from build123d import *

# Parameters (mm, degrees)
SKETCH1_W           = 9.525
SKETCH1_H           = 9.525
BOSS_EXTRUDE1_DEPTH = 5.1816
SKETCH2_R           = 3.175
BOSS_EXTRUDE2_DEPTH = 6.35
BOSS_EXTRUDE3_DEPTH = 0.762
SKETCH4_R           = 1.5875
BOSS_EXTRUDE4_DEPTH = 6.35
CUT_EXTRUDE1_DEPTH  = 4.826
SKETCH6_R           = 0.254
BOSS_EXTRUDE5_DEPTH = 5.969


with BuildPart() as part:
    # Sketch1 → Boss-Extrude1 (new body)
    with BuildSketch(Plane(origin=(0, 0, 0), x_dir=(1, 0, 0), z_dir=(0, 1, 0))):
        Rectangle(SKETCH1_W, SKETCH1_H)
    extrude(amount=-BOSS_EXTRUDE1_DEPTH)

    # Sketch2 → Boss-Extrude2 (add)
    with BuildSketch(Plane(origin=(0, 0, 0), x_dir=(1, 0, 0), z_dir=(0, 1, 0))):
        Circle(SKETCH2_R)
    extrude(amount=BOSS_EXTRUDE2_DEPTH)

    # Sketch3 → Boss-Extrude3 (add)
    with BuildSketch(Plane(origin=(0, 0, 0), x_dir=(1, 0, 0), z_dir=(0, 1, 0))):
        with BuildLine():
            Line((-4.7625, 0.381), (-4.7625, -0.381))
            ThreePointArc((-4.7625, -0.381), (-4.3815, 0), (-4.7625, 0.381))
        make_face()
    extrude(amount=BOSS_EXTRUDE3_DEPTH)

    # Sketch4 → Boss-Extrude4 (add)
    with BuildSketch(Plane(origin=(0, 6.35, 0), x_dir=(1, 0, 0), z_dir=(0, 1, 0))):
        Circle(SKETCH4_R)
    extrude(amount=BOSS_EXTRUDE4_DEPTH)

    # Sketch5 → Cut-Extrude1 (cut)
    with BuildSketch(Plane(origin=(0, 12.7, 0), x_dir=(1, 0, 0), z_dir=(0, 1, 0))):
        with BuildLine():
            Line((-1.371129549, -0.8001), (1.371129549, -0.8001))
            ThreePointArc((1.371129549, -0.8001), (0, -1.5875), (-1.371129549, -0.8001))
        make_face()
    extrude(amount=-CUT_EXTRUDE1_DEPTH, mode=Mode.SUBTRACT)

    # Sketch6 → Boss-Extrude5 (add)
    with BuildSketch(Plane.XZ.offset(5.1816)):
        with Locations((0, 2.54)):
            Circle(SKETCH6_R)
        with Locations((-2.54, -2.54)):
            Circle(SKETCH6_R)
        with Locations((2.54, -2.54)):
            Circle(SKETCH6_R)
    extrude(amount=BOSS_EXTRUDE5_DEPTH)


solid = part.part
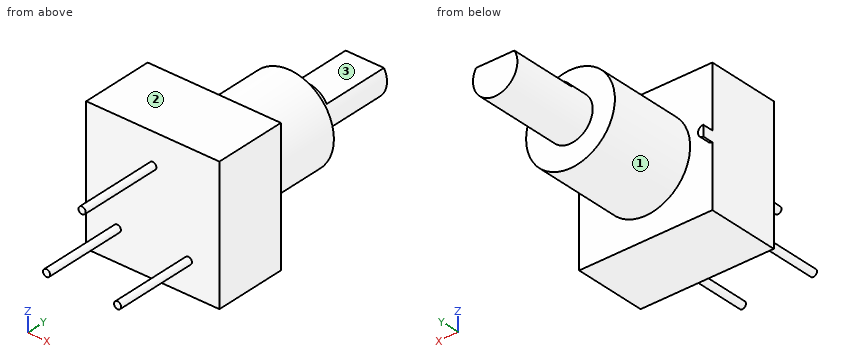
CAD build for the part. Positions are in the model's coordinates, mm. Face numbers are marked on the shaded views. A direction names the side the tool comes from. Coordinates: 2 decimals unless noted, no trailing zeros. Write each loop counter-clockwise with the first axis right and the second up, starting at its lowest first coordinate (ties: lowest second). Pieces come first, ordered by that corner, then holes. Notation, with made-up numbers: M -36.75,-36 L 22.25,-36 A12 ccw 22.25,-18 Z; hole C 13,82.25 d11. An arc over 180 degrees is marked long. Return JSON: item names as keys, results as strings.
Item 1: Slice it at D-D, the plane y = 1.75. Write the cut outline in (x, z) (3 decimals).
Findings below:
{"outline": "C 0,0 d6.35"}
Item 2: Probe line 1 (Y direction, x = -0.75, z = 1); line 2 (Y direction, x = -3, z = 1.75); line 3 (Z direction, x = 0, y = 6) (3 decimals). List the from-to ranges inside material, lowest first. Write a range as from..to.
Findings below:
{"line 1": "y = -5.18..7.87", "line 2": "y = -5.18..0", "line 3": "z = -3.175..3.175"}
Item 3: Slice it at B-B, the plane y = -8.25. Write the cut outline in (x, z).
Findings below:
{"outline": "C -2.54,-2.54 d0.51; C 0,2.54 d0.51; C 2.54,-2.54 d0.51"}
Item 4: Which spindle directions (+Z, -Z, +X, -X, +Y, -Y) get a long thin tool onto all of the face, cutting with end or side? Do the marked faces 1, 2 and 3. Say none if no direction does.
Findings below:
{"face 1": "+Y", "face 2": "+Z, +X, -X, +Y, -Y", "face 3": "+Z, +X, -X, +Y"}
Item 5: Drop flat-ended pins along their axis: pin 1 Ø1.5 at (y, z) = (5.5, -2.5) entering from -X; pin 2 Ø5 at (x, y) = (-1, 3) entering from +Z (3 decimals); pin 3 Ø3 at (x, y) = (0, 11) entering from +Z; pin 4 Ø2 at (y, z) = (-6, 1.5) entering from +X. Give the stop position or say it passes through.
Findings below:
{"pin 1": "stops at x = -2.65", "pin 2": "stops at z = 3.175", "pin 3": "stops at z = 0.8", "pin 4": "stops at x = 4.76"}
